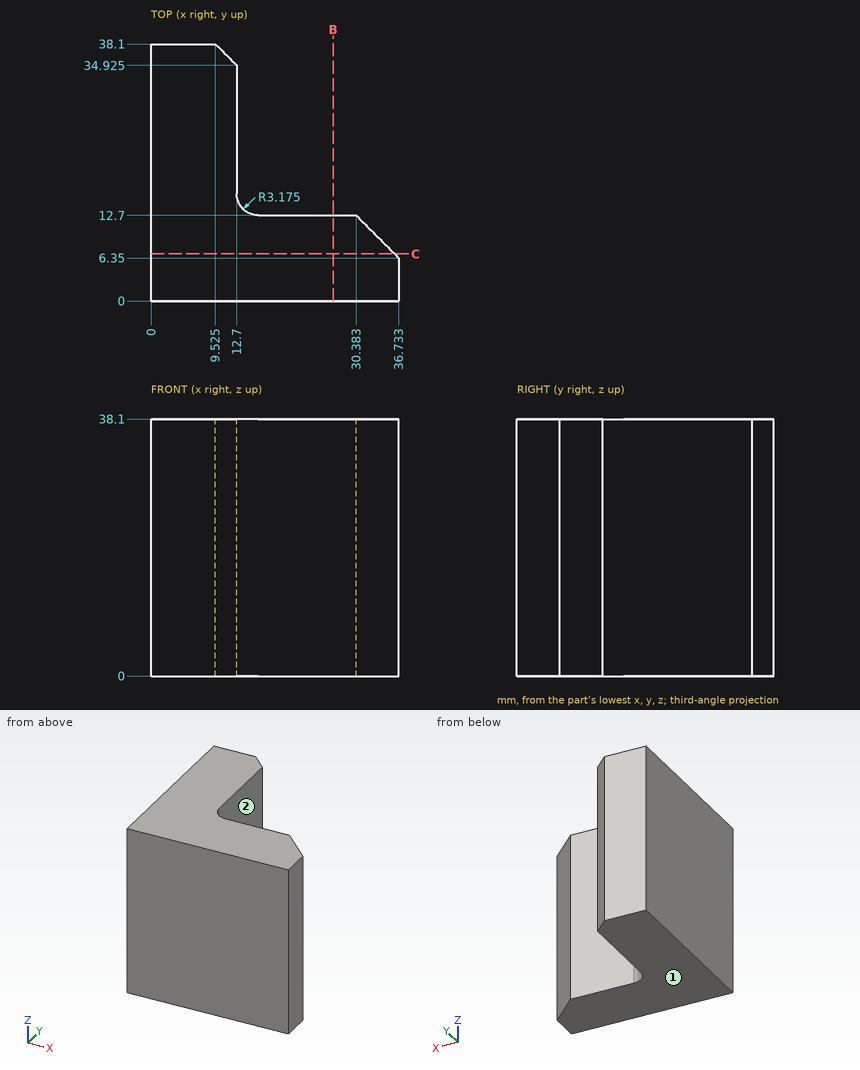
Could you check a few things on this drawing? It's one solid part, dimensions in mm from its lowest x, y, z. A direction names the side the tool comes from. Coordinates: 2 decimals unless noted, no trailing zeros. Write each loop counter-clockwise with the first axis right and the second up, starting at its lowest first coordinate (ties: lowest second). Pieces come first, ordered by that corner, then holes. Notation, with made-up numbers: (87.25, -19) - (144.25, -19) arc R28 cw to (144.25, 18) - close; hole circle Ø5 at (4.25, 81). An arc over 180 degrees is marked (long way). Use one line per item in the form item = value.
1) On a 3-axis mill with a long thin cutter (end or side, diameter ignored), from which of +Z, -Z, +X, -X, +Y, -Y can I reach the whole of each face in a straight line? I mean the marked faces 1 and 2. Say none if no direction works.
Solved:
face_1 = -Z, +X, -X, +Y, -Y
face_2 = +Z, -Z, +X, +Y
2) I'm going to push flat-ended pins straight in: P1, Ø10, axis at x = 19.5, z = 17.5, coming from the +Y side; P2, Ø1.5, axis at y = 33, z = 10.5, coming from the +X side; P3, Ø4.5, axis at x = 25.5, z = 22.5, coming from the +Y side. Where does each tip first touch, or does it pass through?
Solved:
P1 = 13.01
P2 = 12.7
P3 = 12.7
3) I need wall thicknesses on line 1 (Y direction, x = 26, z = 23); line 2 (X direction, y = 35.5, z = 27) (1 decimal). Which ranges of each line are inside material? Lowest first, please.
Solved:
line_1 = 0 to 12.7
line_2 = 0 to 12.1
4) Suppose I cut it at B-B, the plane x = 27. Write out the boundary of the cut face in (y, z), plus the area to 3 significant figures.
Solved:
outline = (0, 0) - (12.7, 0) - (12.7, 38.1) - (0, 38.1) - close
area = 484 mm2
5) Suppose I cut it at C-C, the plane y = 7. Write out the boundary of the cut face in (x, z).
Solved:
outline = (0, 0) - (36.08, 0) - (36.08, 38.1) - (0, 38.1) - close
